```python
from build123d import *

# Parameters (mm, degrees)
BOSS_EXTRUDE1_DEPTH = 2
SKETCH2_R           = 5
CUT_EXTRUDE1_DEPTH  = 4.1


with BuildPart() as part:
    # Sketch1 → Boss-Extrude1 (new body)
    with BuildSketch(Plane.XY):
        with BuildLine():
            Line((-50.768947103, -2.903737712), (-11.597374228, -2.903737712))
            Line((-11.597374228, -2.903737712), (-2.768947103, -11.732164837))
            Line((-2.768947103, -11.732164837), (-2.768947103, -20.903737712))
            ThreePointArc((-2.768947103, -20.903737712), (-5.112092854, -26.560591962), (-10.768947103, -28.903737712))
            Line((-10.768947103, -28.903737712), (-50.768947103, -28.903737712))
            ThreePointArc((-50.768947103, -28.903737712), (-56.425801353, -26.560591962), (-58.768947103, -20.903737712))
            Line((-58.768947103, -20.903737712), (-58.768947103, -10.903737712))
            ThreePointArc((-58.768947103, -10.903737712), (-56.425801353, -5.246883463), (-50.768947103, -2.903737712))
        make_face()
    extrude(amount=BOSS_EXTRUDE1_DEPTH)

    # Sketch2 → Cut-Extrude1 (cut)
    with BuildSketch(Plane(origin=(0, 0, 0), x_dir=(-1, 0, 0), z_dir=(0, 0, -1))):
        with Locations((44.768947103, -15.903737712)):
            Circle(SKETCH2_R)
    extrude(amount=-CUT_EXTRUDE1_DEPTH, mode=Mode.SUBTRACT)


solid = part.part
```
Work out the finished part from the listing and answer in its coordinate system (mm). Round coordinates to 2 decimals unless told otherwise and drop trailing zeros. Order: outer loops, then holes, each group sorted by start corner. A loop starts at its lowest first (then second) coordinate and runs counter-clockwise, first axis right, second up.
Q1. Find the intervals of material crossed by line 1 along Y through (x, z) = (-49, 1.3); line 2 along X through (y, z) = (-18, 0.1); line 3 along X through (y, z) = (-16.75, 1.2), in increasing order.
Solution:
line 1: y = -28.9 to -18.57, -13.24 to -2.9
line 2: x = -58.77 to -49.31, -40.23 to -2.77
line 3: x = -58.77 to -49.7, -39.84 to -2.77
Q2. A cutting plane is placed at C-C, the plane y = -13.25. Determine the outline of the cut face in (x, z).
Solution:
outline: (-58.77, 0) - (-49.01, 0) - (-49.01, 2) - (-58.77, 2) - close; (-40.53, 0) - (-2.77, 0) - (-2.77, 2) - (-40.53, 2) - close
Q3. A cutting plane is placed at B-B, the plane z = 0.3. Determine the outline of the cut face in (x, y), then the cut area to 3 significant figures.
Solution:
outline: (-58.77, -20.9) arc R8 ccw to (-50.77, -28.9) - (-10.77, -28.9) arc R8 ccw to (-2.77, -20.9) - (-2.77, -11.73) - (-11.6, -2.9) - (-50.77, -2.9) arc R8 ccw to (-58.77, -10.9) - close; hole circle Ø10 at (-44.77, -15.9)
area: 1,300 mm2
Q4. The mould has two halves that part along X. Classify faces 1 (the cylindrical face through (-41.084, -12.525, 0.986)), 2 (the flat face through (-7.2, -7.3, 1)), 3 (the flat face through (-30, -16, 0)), 4 (the cylindrical face through (-56.49, -5.31, 0.99)): pulls with the +X half, pulls with the -X half, needs draft (parallel to the pull), parting line crosses it, or undercut.
Solution:
face 1: undercut
face 2: pulls with the +X half
face 3: needs draft
face 4: pulls with the -X half
Q5. A cutting plane is placed at A-A, the plane x = -46.5. Determine the outline of the cut face in (y, z), then the cut area to 3 significant figures.
Solution:
outline: (-28.9, 0) - (-20.59, 0) - (-20.59, 2) - (-28.9, 2) - close; (-11.21, 0) - (-2.9, 0) - (-2.9, 2) - (-11.21, 2) - close
area: 33.2 mm2
Q6. A cutting plane is placed at D-D, the plane y = -9.5. Determine the outline of the cut face in (x, z).
Solution:
outline: (-58.64, 0) - (-5, 0) - (-5, 2) - (-58.64, 2) - close
